Verification items for this drawing (mm, ordinates from the low corner). A direction names the side the tool comes from. Give positions to 0.01 mm unless a question says otherwise; leave off trailing zeros. Loops run counter-clockwise (first coordinate to the right, second up) from the corner with the lowest first, then second, coordinate; pieces in that order, holes last. Notation, with made-up numbers: (-6.5, 63) -> (42.5, 63) arc R19 cw to (42.5, 86) -> close; hole circle Ø3 at (8, 79). An arc over 180 degrees is marked (long way). Answer as a JSON object with one key per item and string values.
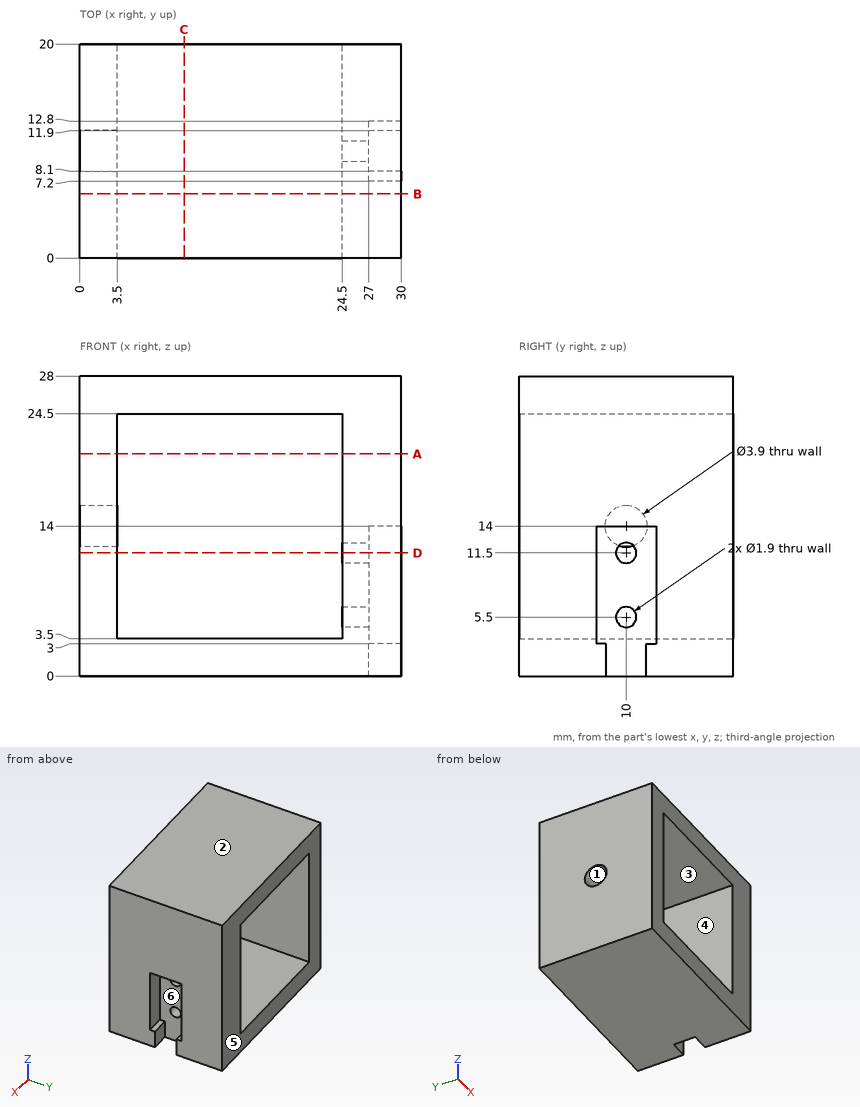
1) Section check C-C on x = 9.75. Record the cut outline in (y, z), plus the area to 3 significant figures.
Geometry check:
{"outline": "(0, 0) -> (20, 0) -> (20, 3.5) -> (0, 3.5) -> close; (0, 24.5) -> (20, 24.5) -> (20, 28) -> (0, 28) -> close", "area": "140 mm2"}
2) Section check B-B on y = 6. Record the cut outline in (x, z).
Geometry check:
{"outline": "(0, 0) -> (30, 0) -> (30, 28) -> (0, 28) -> close; hole (3.5, 3.5) -> (24.5, 3.5) -> (24.5, 24.5) -> (3.5, 24.5) -> close"}
3) Section check D-D on z = 11.5. Record the cut outline in (x, y), plus the area to 3 significant figures.
Geometry check:
{"outline": "(0, 0) -> (3.5, 0) -> (3.5, 20) -> (0, 20) -> close; (24.5, 0) -> (30, 0) -> (30, 7.2) -> (27, 7.2) -> (27, 9.05) -> (24.5, 9.05) -> close; (24.5, 10.95) -> (27, 10.95) -> (27, 12.8) -> (30, 12.8) -> (30, 20) -> (24.5, 20) -> close", "area": "158 mm2"}
4) Depth check by flat-ended pin: P1, Ø1.5, axis at x = 29, z = 7.5, coming from the -Y side; P2, Ø3, axis at y = 10, z = 14, coming from the -X side; P3, Ø3, axis at y = 10, z = 5.5, coming from the +X side. Enter the tip coordinate at first touch or a pass-through.
Geometry check:
{"P1": "stops at y = 0", "P2": "stops at x = 24.5", "P3": "stops at x = 27"}
5) Material ranges on line 1 along Z through (x, y) = (0.95, 10); line 2 along Z through (x, y) = (9, 7.5); line 3 along X through (y, z) = (3.5, 20), recorded low to high. Write a range as from..to.
Geometry check:
{"line 1": "z = 0..12.05, 15.95..28", "line 2": "z = 0..3.5, 24.5..28", "line 3": "x = 0..3.5, 24.5..30"}
6) Section check A-A on z = 20.75. Record the cut outline in (x, y).
Geometry check:
{"outline": "(0, 0) -> (3.5, 0) -> (3.5, 20) -> (0, 20) -> close; (24.5, 0) -> (30, 0) -> (30, 20) -> (24.5, 20) -> close"}
7) Tool access check on the marked faces 1, 2 and 3. Record the directions out of +Z, -Z, +X, -X, +Y, -Y that give a thin tool (end or side, any length) a straight path to the whole face; none if there is none.
Geometry check:
{"face 1": "-X", "face 2": "+Z, +X, -X, +Y, -Y", "face 3": "+Y, -Y"}
8) Draft check along Y on the marked faces 4, 5 and 6. Enter one of: pulls with the +Y half, pulls with the -Y half, needs draft (parallel to the pull), parting line crosses it, or undercut.
Geometry check:
{"face 4": "needs draft", "face 5": "pulls with the +Y half", "face 6": "undercut"}
